```python
from build123d import *

# Parameters (mm, degrees)
F0_W     = 60
F0_H     = 80
F1_DEPTH = 1.6
F2_W     = 25.4
F2_H     = 2.54
F3_DEPTH = 2.54
F4_R     = 0.5
F5_DEPTH = 8


with BuildPart() as f1:
    # F0 (on Top) → F1 (new body)
    with BuildSketch(Plane.XY):
        with Locations((30, 40)):
            Rectangle(F0_W, F0_H)
    extrude(amount=F1_DEPTH)

    # F2 (on face) → F3 (join)
    with BuildSketch(Plane.XY.offset(1.6)):
        with Locations((30, 1.27)):
            Rectangle(F2_W, F2_H)
    extrude(amount=F3_DEPTH)

    # F4 (on face) → F5 (join)
    with BuildSketch(Plane.XZ):
        with Locations((20.157567, 4.14)):
            Circle(F4_R)
        with Locations((22.697567, 4.14)):
            Circle(F4_R)
        with Locations((25.237567, 4.14)):
            Circle(F4_R)
        with Locations((27.777567, 4.14)):
            Circle(F4_R)
        with Locations((30.317567, 4.14)):
            Circle(F4_R)
        with Locations((32.857567, 4.14)):
            Circle(F4_R)
        with Locations((35.397567, 4.14)):
            Circle(F4_R)
        with Locations((37.937567, 4.14)):
            Circle(F4_R)
    extrude(amount=F5_DEPTH)


solid = f1.part
```
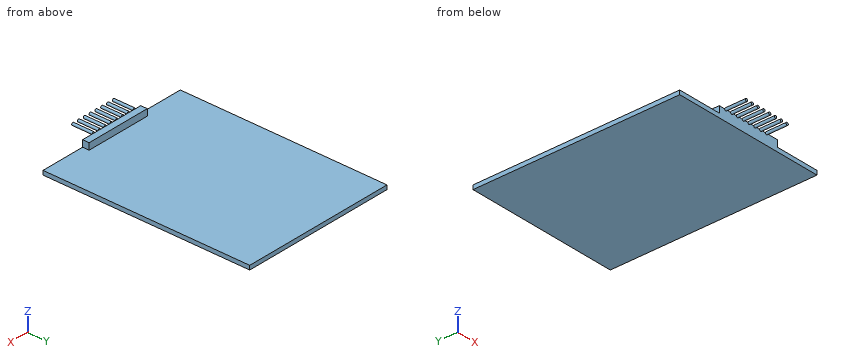
Model file for the job. Use its own axes, mm. Coordinates: 2 decimals unless noted, no trailing zeros. Order: outer loops, then holes, each group sorted by start corner. A loop starts at its lowest first (then second) coordinate and runs counter-clockwise, first axis right, second up. Notation, with made-up numbers: (-8, -40) -> (35, -40) arc R14 cw to (35, -18) -> close; hole circle Ø5 at (69, 18.25). An arc over 180 degrees is marked (long way). Return JSON: item names as keys, results as strings.
Item 1: Pin check, flat tips, straight feed: P1, Ø0.8, axis at x = 28, y = 1.5, coming from the +Z side; P2, Ø0.6, axis at x = 33, z = 4.5, coming from the +Y side; P3, Ø12, axis at x = 13.5, y = 46.5, coming from the +Z side. Stop position of each tip, or through.
Model answer:
{"P1": "stops at z = 4.14", "P2": "stops at y = 0", "P3": "stops at z = 1.6"}
Item 2: Wall check: line 1 along Z through (x, y) = (53, 57.5); line 2 along Y through (x, z) = (40, 4.05); line 3 along Y through (x, z) = (2, 1.4). Give the ranges that are in metal, low to high. Write a range as from..to.
Model answer:
{"line 1": "z = 0..1.6", "line 2": "y = 0..2.54", "line 3": "y = 0..80"}
Item 3: Slice it at A-A (y = 19). Write the cut outline in (x, z).
Model answer:
{"outline": "(0, 0) -> (60, 0) -> (60, 1.6) -> (0, 1.6) -> close"}
